Read the model definition and answer for the solid it produces. Units are mm, in the model's axes. Coordinates: 2 decimals unless noted, no trailing zeros. Loops run counter-clockwise (first coordinate to the right, second up) from the corner with the lowest first, then second, coordinate; pieces in that order, holes last. Notation, with made-up numbers: (83.25, 9.25) -> (127.25, 9.25) arc R30 ccw to (127.25, 33.25) -> close; hole circle Ø5 at (35.5, -19.5). An arc over 180 degrees is marked (long way). Answer in a Markdown table with one row per item.
Autodesk Inventor part; units mm, degrees
ref_plane "YZ Plane" through (0, 0, 0) normal (1, 0, 0) x (0, 1, 0)
ref_plane "XZ Plane" through (0, 0, 0) normal (0, 1, 0) x (-1, 0, 0)
ref_plane "XY Plane" through (0, 0, 0) normal (0, 0, 1) x (1, 0, 0)
sketch "Sketch1" plane through (0, 0, 0) normal (0, 1, 0) x (-1, 0, 0)
  line L0 (0, 0) -> (108.6, 0)
  line L1 (108.6, 0) -> (108.6, -110.4)
  line L2 (108.6, -110.4) -> (0, -110.4)
  line L3 (0, -110.4) -> (0, 0)
  circle A0 centre (12.3, -77.7) radius 6.5
  circle A1 centre (57.3, -77.7) radius 12
  dimension "d0" = 108.6
  dimension "d1" = 110.4
  dimension "d2" = 13
  dimension "d3" = 12.3
  dimension "d4" = 32.7
  dimension "d5" = 24
  dimension "d6" = 45
extrude "Extrusion1" add sketch "Sketch1" along normal blind 9
properties part number "Marco_frontal" material "Aluminum 6061"
1. A cutting plane is placed at B-B on x = -57.3. Give the vertices of the cut face in (y, z).
A:
| item | result |
|---|---|
| outline | (0, -110.4) -> (9, -110.4) -> (9, -89.7) -> (0, -89.7) -> close; (0, -65.7) -> (9, -65.7) -> (9, 0) -> (0, 0) -> close |
2. Find the intervals of material crossed by probe 1 along Z at (x, y) = (-12.3, 7.25); probe 2 along Z at (x, y) = (-57.3, 3); probe 3 along X at (y, z) = (1.5, -75.5), in increasing order.
A:
| item | result |
|---|---|
| probe 1 | z = -110.4 to -84.2, -71.2 to 0 |
| probe 2 | z = -110.4 to -89.7, -65.7 to 0 |
| probe 3 | x = -108.6 to -69.1, -45.5 to -18.42, -6.18 to 0 |
3. The mould has two halves that part along X. Classify faces 1 (the cylindrical face through (-68.746, 4.437, -81.304)), 2 (the flat face through (-54, 4, 0)), 3 (the flat face through (-108.6, 4, -54)): pulls with the +X half, pulls with the -X half, needs draft (parallel to the pull), parting line crosses it, or undercut.
A:
| item | result |
|---|---|
| face 1 | undercut |
| face 2 | needs draft |
| face 3 | pulls with the -X half |
4. A cutting plane is placed at A-A on z = -77.7. Give the vertices of the cut face in (x, y).
A:
| item | result |
|---|---|
| outline | (-108.6, 0) -> (-69.3, 0) -> (-69.3, 9) -> (-108.6, 9) -> close; (-45.3, 0) -> (-18.8, 0) -> (-18.8, 9) -> (-45.3, 9) -> close; (-5.8, 0) -> (0, 0) -> (0, 9) -> (-5.8, 9) -> close |
5. A cutting plane is placed at C-C on y = 5. Give the vertices of the cut face in (x, z).
A:
| item | result |
|---|---|
| outline | (-108.6, -110.4) -> (0, -110.4) -> (0, 0) -> (-108.6, 0) -> close; hole circle Ø24 at (-57.3, -77.7); hole circle Ø13 at (-12.3, -77.7) |
